Autodesk Inventor part; units mm, degrees
ref_plane "YZ Plane" through (0, 0, 0) normal (1, 0, 0) x (0, 1, 0)
ref_plane "XZ Plane" through (0, 0, 0) normal (0, 1, 0) x (-1, 0, 0)
ref_plane "XY Plane" through (0, 0, 0) normal (0, 0, 1) x (1, 0, 0)
sketch "Sketch1" plane through (0, 0, 0) normal (0, 0, 1) x (1, 0, 0)
  line L0 (-150, 110) -> (150, 110)
  line L1 (150, 110) -> (150, -110)
  line L2 (150, -110) -> (-150, -110)
  line L3 (-150, -110) -> (-150, 110)
  line L4 (-150, 110) -> (150, -110) construction
  line L5 (150, 110) -> (-150, -110) construction
  point P0 (0, 0)
  dimension "d0" = 300
  dimension "d1" = 220
extrude "Extrusion1" add sketch "Sketch1" along normal blind 5
fillet "Fillet2" radius 20 4 edges at (-150, 110, 2.5) (-150, -110, 2.5) (150, -110, 2.5) (150, 110, 2.5)
chamfer "Chamfer1" distance 1 angle 45 8 edges at (0, -110, 0) (144.1421, -104.1421, 0) (150, 0, 0) (144.1421, 104.1421, 0) (0, 110, 0) (-144.1421, 104.1421, 0) (-150, 0, 0) (-144.1421, -104.1421, 0)
sketch "Sketch8" plane through (0, 0, 0) normal (0, 0, 1) x (1, 0, 0)
  line L0 (-130, 110) -> (130, 110)
  line L1 (-150, -90) -> (-150, 90)
  point P0 (0, 0)
  point P1 (-140, 37)
  point P2 (-50, 100)
  point P3 (-136, 96)
  dimension "d100" = 14
  dimension "d101" = 14
  dimension "d102" = 10
  dimension "d103" = 10
  dimension "d104" = 100
  dimension "d105" = 73
hole "Hole4" at (-140, 37, 0) at (-50, 100, 0) at (-136, 96, 0) direction (0, 0, 1) diameter 3.4 end through all countersink diameter 7.5 countersink angle 90
mirror "Mirror1" about plane through (0, 0, 0) normal (1, 0, 0) of "Hole4"
mirror "Mirror2" about plane through (0, 0, 0) normal (0, 1, 0) of "Hole4", "Mirror1"
sketch "Sketch9" plane through (0, 0, 0) normal (0, 0, -1) x (-1, 0, 0)
  line L0 (125, -85) -> (-125, -85) construction
  line L1 (-125, -85) -> (-125, 85) construction
  line L2 (-125, 85) -> (125, 85) construction
  line L3 (125, 85) -> (125, -85) construction
  line L4 (150, 90) -> (150, -90)
  line L5 (-130, 110) -> (130, 110)
  point P0 (0, 0)
  point P1 (0, 85)
  point P2 (-125, 0)
  dimension "d106" = 25
  dimension "d107" = 25
hole "Hole5" at (-125, -85, 0) at (125, 85, 0) at (125, -85, 0) at (-125, 85, 0) direction (0, 0, 1) diameter 9 depth 2
sketch "Sketch10" plane through (0, 0, 0) normal (0, 0, -1) x (-1, 0, 0)
  line L0 (-35.7, 71.2) -> (35.7, 71.2) construction
  point P0 (0, 71.2)
  point P1 (0, 0)
  dimension "d115" = 71.2
  dimension "d116" = 71.4
hole "Hole6" at (35.7, 71.2, 0) at (-35.7, 71.2, 0) direction (0, 0, 1) diameter 3.4 end through all countersink diameter 7.5 countersink angle 90
sketch "Sketch11" plane through (0, 0, 0) normal (0, 0, -1) x (-1, 0, 0)
  line L0 (77.9535, 19.5226) -> (115.4377, 53.3631) construction
  line L1 (34.4702, 98.6683) -> (96.6956, 36.4429) construction
  line L2 (-130, 110) -> (130, 110)
  point P0 (0, 0)
  dimension "d124" = 50.5
  dimension "d134" = 87.076
  dimension "d135" = 88
  dimension "d136" = 45
hole "Hole7" at (-77.9535, 19.5226, 0) at (-115.4377, 53.3631, 0) direction (0, 0, 1) diameter 3.4 end through all countersink diameter 7.5 countersink angle 90
sketch "Sketch12" plane through (0, 0, 0) normal (0, 0, -1) x (-1, 0, 0)
  line L0 (-32.5, 90) -> (32.5, 90) construction
  line L1 (32.5, 90) -> (32.5, 45) construction
  line L2 (32.5, 45) -> (-32.5, 45) construction
  line L3 (-32.5, 45) -> (-32.5, 90) construction
  point P0 (0, 0)
  point P1 (0, 45)
  dimension "d137" = 45
  dimension "d138" = 45
  dimension "d139" = 65
hole "Hole8" at (32.5, 90, 0) at (-32.5, 45, 0) at (-32.5, 90, 0) at (32.5, 45, 0) direction (0, 0, 1) diameter 3.4 end through all countersink diameter 7.5 countersink angle 90
equation "\"d107\" = d106"
properties part number "Bottom Plate Sanwa" material "Polycarbonate, Clear"
Check sheet for the modelled part. Datum: model origin and axes. Units: mm. A direction names the side the tool comes from. Round coordinates to 2 decimals unless told otherwise and drop trailing zeros. Answer as CSV lines item,"result". Start each with the question number.
Item 1: Set-up check for faces 4 (the flat face through (-2, 2, 5)), 5 (the flat face through (-125, -85, 2)): record each of +Z, -Z, +X, -X, +Y, -Y from which the full face is reachable in a straight line by a thin tool's end or side.
Item 2: Depth check by flat-ended pin: P1, Ø4, axis at x = 140, y = -37, coming from the -Z side; P2, Ø5.5, axis at x = 125, y = -85, coming from the -Z side. Enter the tip coordinate at first touch or a pass-through.
Item 3: Scan lines: line 1 (X direction, y = 90, z = 3.2); line 2 (Y direction, x = -50, z = 3.75); line 3 (Y direction, x = 125, z = 0.95). Record each from-to range of solid material in increasing order. Write a range as [from, to].
Item 4: Release check for a two-part mould opening along Y. For faces 1 (the conical face through (-143.408, 103.706, 0.174)), 2 (the cylindrical face through (-144.297, -103.986, 3.028)), 3 (the conical face through (-141.785, 36.604, 1.922)) record: +Y half, -Y half, draft (parallel to the pull), parting line (faces both ways), or undercut.
Report:
1,face 4,"+Z, +X, -X, +Y, -Y"
1,face 5,"-Z"
2,P1,"stops at z = 1.75"
2,P2,"stops at z = 2"
3,line 1,"x = [-150, -34.2], [-30.8, 30.8], [34.2, 150]"
3,line 2,"y = [-110, -101.7], [-98.3, 98.3], [101.7, 110]"
3,line 3,"y = [-109.95, -89.5], [-80.5, 80.5], [89.5, 109.95]"
4,face 1,"+Y half"
4,face 2,"-Y half"
4,face 3,"undercut"
